from build123d import *

# Parameters (mm, degrees)
F1_DEPTH      = 3
F2_R          = 1.49999
F4_D          = 1
F5_R          = 2.5
F6_R          = 0.1
F8_DEPTH      = 0.1
F8_DEPTH_BACK = 3.1


# Not quite as in the source:
# - a fillet or chamfer is up to 0.001 mm smaller than in the source, because OpenCascade refuses the exact size


with BuildPart() as f1:
    # F0 (on Front) → F1 (new body)
    with BuildSketch(Plane.XZ):
        with BuildLine():
            Line((0, 5), (0, 0))
            Line((0, 0), (4.6566454311, 0))
            Line((4.6566454311, 0), (4.6566454311, 2))
            ThreePointArc((4.6566454311, 2), (6.3577308128, 3.7010853817), (8.0588161945, 2))
            Line((8.0588161945, 2), (8.0588161945, 0))
            Line((8.0588161945, 0), (9.3132908622, 0))
            Line((9.3132908622, 0), (9.3132908622, 5))
            Line((9.3132908622, 5), (0, 5))
        make_face()
    extrude(amount=F1_DEPTH)

    # F2 (radius 1.5 in the source; OpenCascade refuses exactly that, so slightly less here)
    f2_edges = [f1.edges().sort_by_distance(p)[0] for p in [
        (0, 0, 2.5),
        (0, -3, 2.5),
    ]]
    fillet(f2_edges, radius=F2_R)

    # F4 (through all)
    with Locations(Plane.XY.offset(5)):
        with Locations((1.5, -1.5)):
            Hole(F4_D / 2)

    # F5
    f5_edges = [f1.edges().sort_by_distance(p)[0] for p in [
        (9.313291, -1.5, 5),
    ]]
    fillet(f5_edges, radius=F5_R)

    # F6
    f6_edges = [f1.edges().sort_by_distance(p)[0] for p in [
        (4.15664, -3, 5),
        (8.581058, -3, 4.267767),
        (9.313291, -3, 1.25),
        (9.313291, 0, 1.25),
        (8.581058, 0, 4.267767),
        (4.15664, 0, 5),
    ]]
    fillet(f6_edges, radius=F6_R)

    # F7 (on face) → F8 (join, two sides)
    with BuildSketch(Plane.XZ.offset(3)) as f8_sk:
        with BuildLine():
            Line((3.8816455076, 2), (3.8816455076, 0))
            Line((3.8816455076, 0), (4.6566454311, 0))
            Line((4.6566454311, 0), (4.6566454311, 2))
            ThreePointArc((4.6566454311, 2), (6.3577308128, 3.7010853817), (8.0588161945, 2))
            Line((8.0588161945, 2), (8.0588161945, 0))
            Line((8.0588161945, 0), (8.833816118, 0))
            Line((8.833816118, 0), (8.833816118, 2))
            ThreePointArc((8.833816118, 2), (6.3577308128, 4.4760853052), (3.8816455076, 2))
        make_face()
    extrude(amount=F8_DEPTH)
    extrude(f8_sk.sketch, amount=-F8_DEPTH_BACK)


solid = f1.part
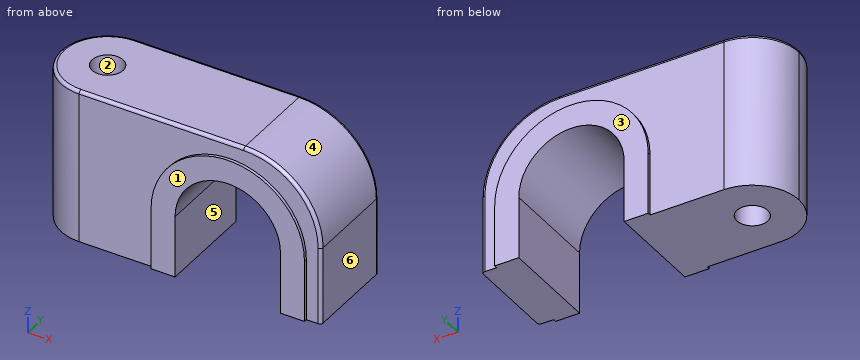
Model file for the job. Use its own axes, mm. Face numbers are marked on the shaded views. A direction names the side the tool comes from. Round coordinates to 2 decimals unless told otherwise and drop trailing zeros. Order: outer loops, then holes, each group sorted by start corner. A loop starts at its lowest first (then second) coordinate and runs counter-clockwise, first axis right, second up. Notation, with made-up numbers: M 48.25,48 L 95.25,48 A24 ccw 95.25,69 Z; hole C 18,-4.5 d7. An arc over 180 degrees is marked long. Write each question's results on one line, items separated by ' | '. Start each with the question number.
(1) Probe probe 1 along Y at (x, z) = (1.5, 3.6); probe 2 along X at (y, z) = (-1.8, 2.6); probe 3 along X at (y, z) = (-1.2, 1.05). List the from-to ranges inside material, lowest first. Write a range as from..to.
(2) Saw through at A-A, the plane z = 0.35. State how many separate pieces and enclosed holes the cut face has, then the cut area to 3 significant figures.
(3) Saw through at C-C, the plane x = 5. Give the cut face in (y, z), then the cut area to 3 significant figures.
(4) Which spindle directions (+Z, -Z, +X, -X, +Y, -Y) get a long thin tool onto all of the face, cutting with end or side? Do the marked faces 5 and 6. Say none if no direction does.
(5) Two-plate mould, pull along Y, no slides. Class the marked faces 1, 2, 3 and 4: pulls with the +Y half, pulls with the -Y half, needs draft (parallel to the pull), parting line crosses it, or undercut.
(6) Saw through at B-B, the plane x = 1.75. Give the cut face in (y, z).
(7) Drop a flat-ended pin along its axis: pin 1 (1.5 mm diameter, centred on x = 5, z = 2.5, fed in from +Y). Give the stop position or say it passes through.
Established:
1) probe 1: y = -3..-2, -1..0 | probe 2: x = 0.03..1.1, 1.9..4.77, 7.95..9.31 | probe 3: x = 0.03..1.1, 1.9..4.66, 8.06..9.31
2) separate pieces: 2 | enclosed holes: 1 | area: 16.3 mm^2
3) outline: M -3.1,3.02 L 0.1,3.02 L 0.1,4.07 L 0,4.07 L 0,4.9 A0.1 ccw -0.1,5 L -2.9,5 A0.1 ccw -3,4.9 L -3,4.07 L -3.1,4.07 Z | area: 6.13 mm^2
4) face 5: -Z, +Y, -Y | face 6: +Z, -Z, +X, +Y, -Y
5) face 1: pulls with the -Y half | face 2: undercut | face 3: pulls with the +Y half | face 4: needs draft
6) outline: M -3,0 L -1.93,0 L -1.93,5 L -2.9,5 A0.1 ccw -3,4.9 Z; M -1.07,0 L 0,0 L 0,4.9 A0.1 ccw -0.1,5 L -1.07,5 Z
7) pin 1: stops at y = 0.1
